Read the model definition and answer for the solid it produces. Units are mm, in the model's axes. A direction names the side the tool comes from. Coordinates: 2 decimals unless noted, no trailing zeros. Write each loop counter-clockwise with the first axis right and the second up, starting at its lowest first coordinate (ties: lowest second). Pieces come first, ordered by that corner, then holes.
(1) Straight lines are drawn through the part: line 1 along Y through (x, z) = (-12.5, -18); line 2 along X through (y, z) = (-151.5, -1.5); line 3 along Z through (x, y) = (3, -236.5). For each, find the intervals that lie inside material, in ascending order.
(2) Determine the mould class of faces 6 (the flat face through (-11, -676, 26.178)), 7 (the flat face through (-61.508, -676, 0)), 8 (the flat face through (-11, -624, 0.778)) for opening direction X: pulls with the +X half, pulls with the -X half, needs draft (parallel to the pull), parting line crosses it, or undercut.
(3) Given pin 1 (1.5 mm diameter, centred on y = -152.5, z = 20.5, fed in from -X); pin 2 (1.5 mm diameter, centred on y = -353.5, z = 5.5, fed in from +X); pin 3 (10 mm diameter, centred on x = -6, y = -629.5, fed in from -Z), each flat-ended and moving along its own axis, determine where each tip first touches the part or whether it passes through.
(4) The part is cut by section D-D, the plane x = -11.5. Determine the outline of the cut face in (y, z).
(5) The part is cut by section C-C, the plane z = -14.5. Determine the outline of the cut face in (x, y), and give its area (3 significant figures).
(6) The part is cut by section B-B, the plane x = -247. Determine the outline of the cut face in (y, z), and give its area (3 significant figures).
(7) Which of the six approach directions +Z, -Z, +X, -X, +Y, -Y give full straight-line access (tool end or side, diameter ignored) to faces 1 (the cylindrical face through (-12.949, -639.897, -12.1)), 2 (the flat face through (-11, -1326, -24.622)), 3 (the flat face through (156, -1069, -24.622)), 4 (the flat face through (-11, -419, -24.622)), 5 (the flat face through (-174, -1069, -24.622))?
(8) The part is cut by section A-A, the plane y = -1111. Determine the outline of the cut face in (x, z).
```python
from build123d import *

# Parameters (mm, degrees)
F0_W     = 101.6
F0_H     = 50.8
F1_DEPTH = 1371.6
F2_R     = 16.7386
F3_DEPTH = 25.4
F4_W     = 558.8
F4_H     = 431.8
F5_DEPTH = 6.35


with BuildPart() as f1:
    # F0 (on Front) → F1 (new body)
    with BuildSketch(Plane.XZ):
        with Locations((-10.707563, 0.777875)):
            Rectangle(F0_W, F0_H)
    extrude(amount=F1_DEPTH)

    # F2 (on face) → F3 (cut)
    with BuildSketch(Plane(origin=(0, 0, -24.622125), x_dir=(1, 0, 0), z_dir=(0, 0, -1))):
        with Locations((-10.770437, 623.300626)):
            Circle(F2_R)
    extrude(amount=-F3_DEPTH, mode=Mode.SUBTRACT)

    # F4 (on face) → F5 (join)
    with BuildSketch(Plane(origin=(0, 0, -24.622125), x_dir=(1, 0, 0), z_dir=(0, 0, -1))):
        with Locations((-4.258305, 1066.069934)):
            Rectangle(F4_W, F4_H)
    extrude(amount=F5_DEPTH)


solid = f1.part
```
Computed:
1. line 1: y = -1371.6 to -639.95, -606.65 to 0
1. line 2: x = -61.51 to 40.09
1. line 3: z = -24.62 to 26.18
2. face 6: needs draft
2. face 7: pulls with the -X half
2. face 8: undercut
3. pin 1: stops at x = -61.51
3. pin 2: stops at x = 40.09
3. pin 3: stops at z = 0.78
4. outline: (-1371.6, -24.62) - (-1281.97, -24.62) - (-1281.97, -30.97) - (-850.17, -30.97) - (-850.17, -24.62) - (-640.02, -24.62) - (-640.02, 0.78) - (-606.58, 0.78) - (-606.58, -24.62) - (0, -24.62) - (0, 26.18) - (-1371.6, 26.18) - close
5. outline: (-61.51, -1371.6) - (40.09, -1371.6) - (40.09, 0) - (-61.51, 0) - close; hole circle Ø33.48 at (-10.77, -623.3)
5. area: 138,000 mm2
6. outline: (-1281.97, -30.97) - (-850.17, -30.97) - (-850.17, -24.62) - (-1281.97, -24.62) - close
6. area: 2,740 mm2
7. face 1: -Z
7. face 2: -Z, +X, -X, -Y
7. face 3: +Z, +X, +Y, -Y
7. face 4: -Z, +X, -X, +Y
7. face 5: +Z, -X, +Y, -Y
8. outline: (-283.66, -30.97) - (275.14, -30.97) - (275.14, -24.62) - (40.09, -24.62) - (40.09, 26.18) - (-61.51, 26.18) - (-61.51, -24.62) - (-283.66, -24.62) - close
